Autodesk Inventor part; units mm, degrees
ref_plane "YZ Plane" through (0, 0, 0) normal (1, 0, 0) x (0, 1, 0)
ref_plane "XZ Plane" through (0, 0, 0) normal (0, 1, 0) x (-1, 0, 0)
ref_plane "XY Plane" through (0, 0, 0) normal (0, 0, 1) x (1, 0, 0)
sketch "スケッチ1" plane through (0, 0, 0) normal (0, 0, 1) x (1, 0, 0)
  circle A0 centre (0, 0) radius 6
  circle A1 centre (0, 0) radius 3
  dimension "d0" = 12
  dimension "d1" = 6
extrude "押し出し1" add sketch "スケッチ1" along normal blind 1
sketch "スケッチ2" plane through (0, 0, 1) normal (0, 0, 1) x (1, 0, 0)
  circle A0 centre (0, 0) radius 6
  circle A1 centre (0, 0) radius 3
  circle A2 centre (0, 0) radius 4
  dimension "d4" = 8
extrude "押し出し2" add sketch "スケッチ2" along normal blind 5 contours A2
chamfer "面取り1" distance 0.5 angle 45 1 edges at (-4, 0, 6)
properties part number "オイレスw5f6-10a" material "アセタール樹脂、黒"
Model file for the job. Use its own axes, mm. Coordinates: 2 decimals unless noted, no trailing zeros. Order: outer loops, then holes, each group sorted by start corner. A loop starts at its lowest first (then second) coordinate and runs counter-clockwise, first axis right, second up. Notation, with made-up numbers: (-20, 75) -> (28, 75) arc R9 cw to (28, 84) -> close; hole circle Ø1 at (55, 44). An arc over 180 degrees is marked (long way). Return JSON: item names as keys, results as strings.
Item 1: Mould opens along X. For faces 1 (the face through (-1.42, -3.92, 1)), 2 (the face through (-0.867, 3.905, 3.218)), 3 (the face through (-3, 0, 3)) say: pulls with the +X half, pulls with the -X half, needs draft (parallel to the pull), parting line crosses it, or undercut.
Model answer:
{"face 1": "needs draft", "face 2": "parting line crosses it", "face 3": "undercut"}
Item 2: Pin check, flat tips, straight feed: P1, Ø3.5, axis at x = 0, y = 0, coming from the -Z side; P2, Ø1, axis at y = 0.5, z = 2.5, coming from the -X side; P3, Ø1, axis at y = 2.5, z = 4.5, coming from the +X side. Stop position of each tip, or through.
Model answer:
{"P1": "passes through", "P2": "stops at x = -4", "P3": "stops at x = 3.46"}
Item 3: Slice it at C-C (z = 2.65). Write the cut outline in (x, y).
Model answer:
{"outline": "circle Ø8 at (0, 0); hole circle Ø6 at (0, 0)"}
Item 4: Slice it at A-A (y = 0). Write the cut outline in (x, z), then the cut area to 4 significant figures.
Model answer:
{"outline": "(-6, 0) -> (-3, 0) -> (-3, 6) -> (-3.5, 6) -> (-4, 5.5) -> (-4, 1) -> (-6, 1) -> close; (3, 0) -> (6, 0) -> (6, 1) -> (4, 1) -> (4, 5.5) -> (3.5, 6) -> (3, 6) -> close", "area": "15.75 mm²"}
Item 5: Wall check: line 1 along Y through (x, z) = (0, 4.1); line 2 along X through (y, z) = (-2.25, 4.2); line 3 along X through (y, z) = (-1, 0.35). Give the ranges that are in metal, low to high. Write a range as from..to.
Model answer:
{"line 1": "y = -4..-3, 3..4", "line 2": "x = -3.31..-1.98, 1.98..3.31", "line 3": "x = -5.92..-2.83, 2.83..5.92"}
